Autodesk Fusion 360 part; units mm, degrees
sketch "Sketch1" plane through (0, 0, 0) normal (0, 0, 1) x (1, 0, 0)
  line L0 (23.6957, -0.0182) -> (23.6957, -10.0069)
  line L1 (-0.0543, -10.0069) -> (23.6957, -10.0069)
  line L2 (17.7267, -0.0264) -> (17.7267, -5.0176)
  line L3 (-0.0543, -5.0176) -> (17.7267, -5.0176)
  line L4 (5.1457, -10.0069) -> (5.1457, -5.0176)
  line L5 (17.7267, -0.0264) -> (16.3734, 1.4275)
  line L6 (17.5959, 2.993) -> (16.3734, 1.4275)
  line L7 (23.6957, -0.0182) -> (22.197, -0.0182)
  line L8 (23.6957, -0.0182) -> (17.7267, -1.5064)
  line L9 (-0.0543, -5.0176) -> (-0.0543, -10.0069)
  line L10 (17.5959, 2.993) -> (22.197, 2.993)
  line L11 (22.197, -0.0182) -> (22.197, 2.993)
  line L12 (23.6957, -0.0182) -> (22.197, -0.0182) construction
  line L13 (17.7267, -5.0176) -> (23.6957, -5.0125)
  line L14 (15.6957, -5.0176) -> (15.6957, -10.0069)
  line L15 (20.6957, -5.0176) -> (20.6957, -10.0069)
  line L16 (17.7267, -2.522) -> (23.6957, -2.522)
  point P0 (17.7267, -0.0264)
  point P1 (5.1457, -10.0069)
  dimension "latch_width" = 5.969
  dimension "d8" = 5.2
  dimension "d16" = 14
  dimension "d26" = 3
  dimension "d27" = 5
  dimension "d41" = 23.75
extrude "Extrude4" add sketch "Sketch1" along normal blind 3.4 makes body 1
extrude "Extrude9" add sketch "Sketch1" against normal blind 3 contours L0 L2 L8 L16 | L0 L2 L13 L16 | L0 L1 L3 L13 L14 | L1 L3 L4 L14 | L1 L3 L4 L9 bodies 1
extrude "Extrude5" add sketch "Sketch1" along normal blind 11.7 contours L0 L2 L8 L16 bodies 1
extrude "Extrude6" add sketch "Sketch1" along normal blind 9.4 contours L0 L1 L3 L13 L14 bodies 1
sketch "Sketch2" plane through (23.6957, 0, 0) normal (1, 0, 0) x (0, 1, 0)
  line L0 (-0.0182, 0) -> (-0.0182, 3.4)
  line L1 (-0.0182, 3.4) -> (-0.0182, 11.7)
  line L2 (-0.0182, 11.7) -> (-2.522, 11.7)
  line L3 (-2.522, 11.7) -> (-2.522, 3.4)
  line L4 (-2.522, 3.4) -> (-5.0125, 3.4)
  line L5 (-5.0125, 3.4) -> (-5.0125, 9.4)
  line L6 (-5.0125, 9.4) -> (-10.0069, 9.4)
  line L7 (-10.0069, 9.4) -> (-10.0069, -3)
  line L8 (-5.0125, 3.4) -> (-10.0069, 3.4)
  line L9 (-10.0069, 3.4) -> (-10.0069, 6.4)
  line L10 (-10.0069, 6.4) -> (-5.0125, 6.4)
  line L11 (-5.0125, 6.4) -> (-5.0125, 3.4)
  line L12 (-10.0069, -3) -> (-0.0182, -3)
  line L13 (-0.0182, -3) -> (-0.0182, 0)
  dimension "d34" = 3
extrude "Extrude7" cut sketch "Sketch2" against normal blind 3 contours L5 L7 L8 L9 L10 L11 bodies 1
mirror "Mirror1" about plane through (-0.0543, -5.0176, 0) normal (-1, 0, 0) of bodies 1 makes body 2
extrude "Extrude8" add 1 faces at (-0.0543, -8.3438, 1.2667) along direction (-1, 0, 0) blind 2 on bodies 1 bodies 1 2
equation "usbconn_width = 10.4 mm"
equation "usbconn_height = 8.3 mm"
equation "d8 = usbconn_width / 2"
equation "slot_height = 3.4 mm"
equation "d28 = slot_height"
equation "d30 = slot_height + usbconn_height"
equation "d32 = slot_height + 6 mm"
equation "d41 = width"
equation "width = 23.75 mm"
For this review, take the finished solid that the model builds, in its own axes (mm). A direction names the side the tool comes from. Round coordinates to 2 decimals unless told otherwise and drop trailing zeros. Loops run counter-clockwise (first coordinate to the right, second up) from the corner with the lowest first, then second, coordinate; pieces in that order, holes last.
(1) Wall thickness on line 1 along X through (y, z) = (-4, 1.75); line 2 along X through (y, z) = (-9, 5.75); line 3 along Z through (x, y) = (20, -4.75): over which ranges is each line inside the solid? List them lowest first.
Returned:
line 1: x = -23.8 to -17.84, 17.73 to 23.7
line 2: x = -20.8 to -15.8, 15.7 to 20.7
line 3: z = -3 to 3.4
(2) We need section D-D (y = -7.75). Give the boundary of the cut face in (x, z), plus the area to 3 significant figures.
Returned:
outline: (-23.8, -3) - (23.7, -3) - (23.7, 3.4) - (20.7, 3.4) - (20.7, 6.4) - (23.7, 6.4) - (23.7, 9.4) - (15.7, 9.4) - (15.7, 3.4) - (-15.8, 3.4) - (-15.8, 9.4) - (-23.8, 9.4) - (-23.8, 6.4) - (-20.8, 6.4) - (-20.8, 3.4) - (-23.8, 3.4) - close
area: 382 mm2
(3) We need section B-B (y = -4.5). Give the boundary of the cut face in (x, z).
Returned:
outline: (-23.8, -3) - (-17.84, -3) - (-17.84, 3.4) - (-23.8, 3.4) - close; (17.73, -3) - (23.7, -3) - (23.7, 3.4) - (17.73, 3.4) - close
(4) We need section A-A (z = 10.5). Give the boundary of the cut face in (x, y).
Returned:
outline: (-23.8, -2.52) - (-17.84, -2.52) - (-17.84, -1.51) - (-23.8, -0.02) - close; (17.73, -2.52) - (23.7, -2.52) - (23.7, -0.02) - (17.73, -1.51) - close
(5) Tool access review of faces 5 (the flat face through (23, -0.018, 2)), 6 (the flat face through (20.753, -0.752, 7.492)), 7 (the flat face through (-23, -0.018, 2)), 8 (the flat face through (22, -8, 6.4)): name each direction out of +Z, -Z, +X, -X, +Y, -Y from which nothing blocks a thin tool from reaching the whole face with its end or side.
Returned:
face 5: +Z, -Z, +X, +Y
face 6: +Z, +Y
face 7: +Z, -Z, -X, +Y
face 8: +X, -Y
(6) We need section C-C (z = 5.25). Give the boundary of the cut face in (x, y).
Returned:
outline: (-23.8, -2.52) - (-17.84, -2.52) - (-17.84, -1.51) - (-23.8, -0.02) - close; (-20.8, -10.01) - (-15.8, -10.01) - (-15.8, -5.02) - (-17.84, -5.02) - (-20.8, -5.02) - close; (15.7, -10.01) - (20.7, -10.01) - (20.7, -5.02) - (17.73, -5.02) - (15.7, -5.02) - close; (17.73, -2.52) - (23.7, -2.52) - (23.7, -0.02) - (17.73, -1.51) - close
(7) Mouldability with a two-part tool opening along Z and no side actions: class faces 1 (the flat face through (0, -10.007, 2)), 2 (the flat face through (20, -7, 9.4)), 3 (the flat face through (-22, -7, 6.4)), 4 (the flat face through (-22, -5, 3.4)) as released by +Z, released by -Z, zero draft, split by the parting line, or undercut.
Returned:
face 1: zero draft
face 2: released by +Z
face 3: undercut
face 4: undercut
(8) Clearance check with flat-ended pins moving along their axes: P1, Ø6, axis at x = -7, z = 2, coming from the +Y side; P2, Ø2.5, axis at x = -19.5, y = -8, coming from the +Z side; P3, Ø4, axis at x = -1.5, y = -8, coming from the +Z side; P4, Ø4, axis at x = 2.5, y = -4.5, coming from the -Z side. State where each tip first meets the part, or that it passes through.
Returned:
P1: stops at y = -5.02
P2: stops at z = 9.4
P3: stops at z = 3.4
P4: stops at z = -3
